```python
from build123d import *

# Parameters (mm, degrees)
F0_W     = 132.08
F0_H     = 50.8
F1_DEPTH = 25.4
F2_W     = 38.1
F2_H     = 31.75
F3_DEPTH = 25.4
F4_DEPTH = 25.4


with BuildPart() as f1:
    # F0 (on Top) → F1 (new body)
    with BuildSketch(Plane.XY):
        with Locations((-82.06671, 36.546972)):
            Rectangle(F0_W, F0_H)
    extrude(amount=F1_DEPTH)

    # F2 (on face) → F3 (join)
    with BuildSketch(Plane.XY.offset(25.4)):
        with Locations((-101.147438, 67.928043)):
            Rectangle(F2_W, F2_H)
    extrude(amount=F3_DEPTH)

    # F2 (on face) → F4 (join)
    with BuildSketch(Plane.XY.offset(25.4)):
        with Locations((-101.147438, 67.928043)):
            Rectangle(F2_W, F2_H)
    extrude(amount=F4_DEPTH)


solid = f1.part
```
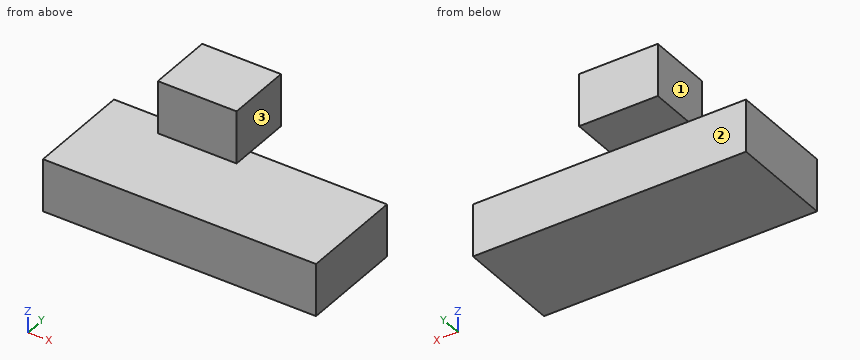
Verification items for the finished model (mm, model axes). Face numbers are marked on the shaded views. A direction names the side the tool comes from. Coordinates: 2 decimals unless noted, no trailing zeros. Write each loop counter-clockwise with the first axis right and the second up, starting at its lowest first coordinate (ties: lowest second). Pieces come first, ordered by that corner, then holes. Notation, with made-up numbers: M 23,46 L 69,46 A17 cw 69,54 Z; hole C -26,54.5 d3. An arc over 180 degrees is marked long. Answer as a JSON object with one key per item and string values. Group by question number.
(1) Cross-section at A-A, the plane x = -116. Record the cut outline in (y, z), and give its area (3 significant figures).
(2) Gauge pin test, flat ends, axial feed: pin 1 (11 mm diameter, centred on x = -97, y = 70.5, fed in from -Z); pin 2 (12.5 mm diameter, centred on y = 69.5, z = 44, fed in from +X); pin 3 (8 mm diameter, centred on y = 25, z = 31, fed in from -X); pin 4 (20.5 mm diameter, centred on y = 72.5, z = 43.5, fed in from -X). Record the tip position at first contact, or that the pin passes through.
(3) Cross-section at D-D, the plane x = -66. Record the cut outline in (y, z).
(4) Tool access check on the marked faces 1, 2 and 3. Record the directions out of +Z, -Z, +X, -X, +Y, -Y that give a thin tool (end or side, any length) a straight path to the whole face; none if there is none.
(5) Cross-section at C-C, the plane z = 32.5. Record the cut outline in (x, y).
(6) Cross-section at B-B, the plane y = 56.5. Record the cut outline in (x, z).
(7) Material ranges on line 1 (Y direction, x = -119, z = 25.5); line 2 (Z direction, x = -32, y = 41.5); line 3 (Z direction, x = -115, y = 64), recorded low to high.
Reply:
{
 "1": {"outline": "M 11.15,0 L 61.95,0 L 61.95,25.4 L 83.8,25.4 L 83.8,50.8 L 52.05,50.8 L 52.05,25.4 L 11.15,25.4 Z", "area": "2,100 mm²"},
 "2": {"pin 1": "z = 25.4", "pin 2": "x = -82.1", "pin 3": "through", "pin 4": "x = -120.2"},
 "3": {"outline": "M 11.15,0 L 61.95,0 L 61.95,25.4 L 11.15,25.4 Z"},
 "4": {"face 1": "+Z, -X, +Y, -Y", "face 2": "-Z, +X, -X, +Y", "face 3": "+Z, +X, +Y, -Y"},
 "5": {"outline": "M -120.2,52.05 L -82.1,52.05 L -82.1,83.8 L -120.2,83.8 Z"},
 "6": {"outline": "M -148.11,0 L -16.03,0 L -16.03,25.4 L -82.1,25.4 L -82.1,50.8 L -120.2,50.8 L -120.2,25.4 L -148.11,25.4 Z"},
 "7": {"line 1": "52.05 to 83.8", "line 2": "0 to 25.4", "line 3": "25.4 to 50.8"}
}
